Print and shaded views of the part. All mm, measured from the part's lowest x, y and z. Round coordinates to 2 decimals unless told otherwise and drop trailing zeros. Loops run counter-clockwise (first coordinate to the right, second up) from the corner with the lowest first, then second, coordinate; pieces in that order, holes last. Notation, with made-up numbers: (54, 50) - (67, 50) arc R18 ccw to (67, 59) - close; hole circle Ø6 at (22.5, -33). An arc over 180 degrees is marked (long way). Use one line per item in the form item = value. Start each with the question number.
Q1. Pin check, flat tips, straight feed: pin 1 (2 mm diameter, centred on x = 9.5, y = 12.5, fed in from -Z); pin 2 (8 mm diameter, centred on x = 11, y = 12, fed in from +Z); pin 3 (8 mm diameter, centred on y = 9.5, z = 13.5, fed in from +X). Stop position of each tip, or through.
Q2. Saw through at C-C (y = 6). Give the cut face in (x, z), then the cut area to 3 significant figures.
Q3. Saw through at D-D (z = 6). Give the cut face in (x, y), then the cut area to 3 significant figures.
Q4. Saw through at B-B (x = 20). Give the cut face in (y, z), then the cut area to 3 significant figures.
Q5. Drill centre lines: line 1 (Y direction, x = 3.5, z = 30.5); line 2 (Z direction, x = 20, y = 5.5); line 3 (X direction, y = 14.5, z = 20). Where is each one in solid material? Low to high.
Q6. Saw through at A-A (z = 20). Give the cut face in (x, y), then the cut area to 3 significant figures.
Q7. Mould opens along Y. For the marked faces 1, 2, 3 and 4 say: released by +Y, released by -Y, zero draft, split by the parting line, or undercut.
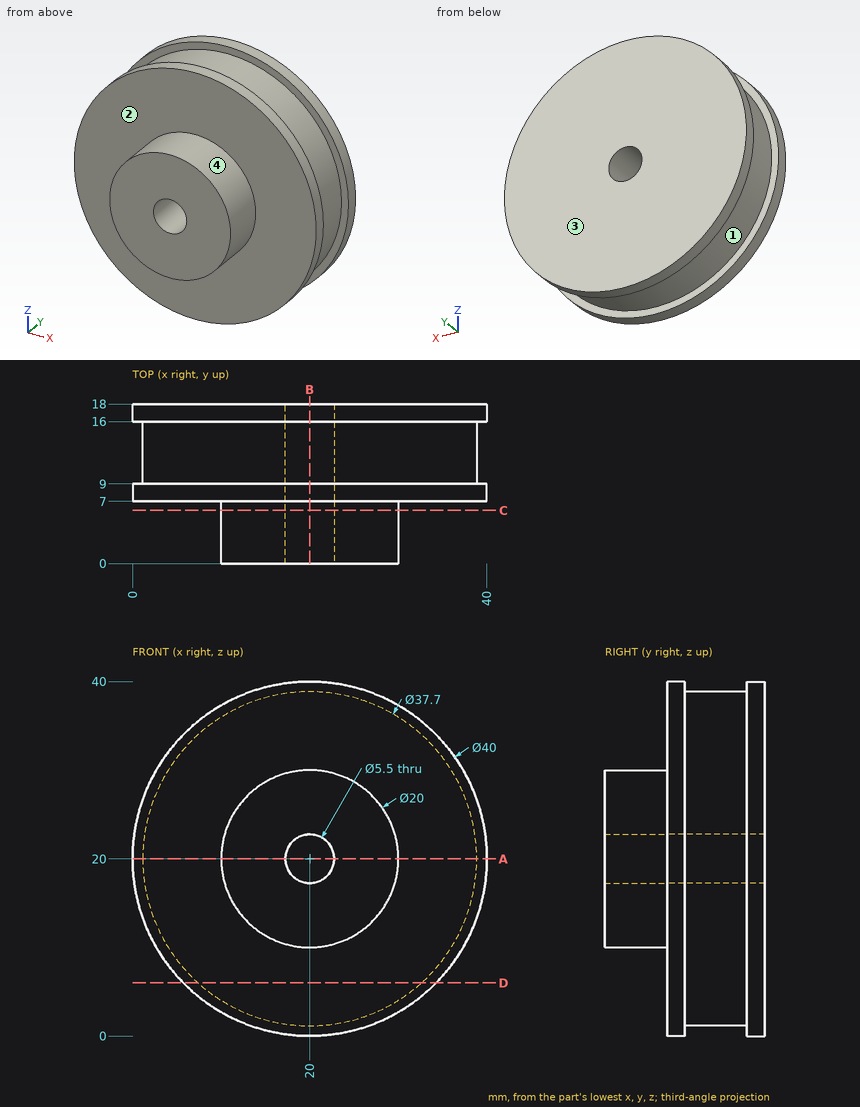
Report:
q1.pin_1 = 3.72
q1.pin_2 = 38.96
q1.pin_3 = 39.84
q2.outline = circle Ø20 at (20, 20); hole circle Ø5.5 at (20, 20)
q2.area = 290 mm²
q3.outline = (5.72, 7) - (34.28, 7) - (34.28, 9) - (32.62, 9) - (32.62, 16) - (34.28, 16) - (34.28, 18) - (5.72, 18) - (5.72, 16) - (7.38, 16) - (7.38, 9) - (5.72, 9) - close
q3.area = 291 mm²
q4.outline = (0, 10) - (7, 10) - (7, 0) - (9, 0) - (9, 1.15) - (16, 1.15) - (16, 0) - (18, 0) - (18, 17.25) - (0, 17.25) - close; (0, 22.75) - (18, 22.75) - (18, 40) - (16, 40) - (16, 38.85) - (9, 38.85) - (9, 40) - (7, 40) - (7, 30) - (0, 30) - close
q4.area = 465 mm²
q5.line_1 = 7 to 9, 16 to 18
q5.line_2 = 10 to 17.25, 22.75 to 30
q5.line_3 = 1.15 to 17.25, 22.75 to 38.85
q6.outline = (0, 7) - (10, 7) - (10, 0) - (17.25, 0) - (17.25, 18) - (0, 18) - (0, 16) - (1.15, 16) - (1.15, 9) - (0, 9) - close; (22.75, 0) - (30, 0) - (30, 7) - (40, 7) - (40, 9) - (38.85, 9) - (38.85, 16) - (40, 16) - (40, 18) - (22.75, 18) - close
q6.area = 465 mm²
q7.face_1 = undercut
q7.face_2 = released by -Y
q7.face_3 = released by +Y
q7.face_4 = zero draft
